from build123d import *

# Parameters (mm, degrees)
F0_R     = 8.5
F1_DEPTH = 2.75
F2_R     = 3.83
F3_DEPTH = 3.6
F4_R     = 2.1875
F5_DEPTH = 3.2
F6_R     = 0.5


with BuildPart() as f1:
    # F0 (on Top) → F1 (new body)
    with BuildSketch(Plane.XY):
        Circle(F0_R)
    extrude(amount=F1_DEPTH)

    # F2 (on face) → F3 (join)
    with BuildSketch(Plane.XY.offset(2.75)):
        Circle(F2_R)
    extrude(amount=F3_DEPTH)

    # F4 (on face) → F5 (cut)
    with BuildSketch(Plane.XY.offset(6.35)):
        Circle(F4_R)
    extrude(amount=-F5_DEPTH, mode=Mode.SUBTRACT)

    # F6
    f6_edges = [f1.edges().sort_by_distance(p)[0] for p in [
        (-8.5, 0, 0),
    ]]
    fillet(f6_edges, radius=F6_R)


solid = f1.part
Model file for the job. Use its own axes, mm. A direction names the side the tool comes from. Coordinates: 2 decimals unless noted, no trailing zeros. Loops run counter-clockwise (first coordinate to the right, second up) from the corner with the lowest first, then second, coordinate; pieces in that order, holes last. Notation, with made-up numbers: (-21.5, 81.25) -> (13.5, 81.25) arc R14 ccw to (13.5, 106.25) -> close; hole circle Ø5 at (61, 57). An arc over 180 degrees is marked (long way). Use one line per item in the form item = value. Start each with the question number.
(1) Probe probe 1 along Y at (x, z) = (0, 4.1); probe 2 along Z at (x, y) = (-2.75, 6.25); probe 3 along X at (y, z) = (1.5, 3.75). List the from-to ranges inside material, lowest first. Write a range as from..to.
(2) Tool access for faces 4 (the flat face through (0, 0, 0)), 5 (the flat face through (4, -2, 2.75)): list every direction of +Z, -Z, +X, -X, +Y, -Y with a clear straight run to the whole face (end or side of a thin tool).
(3) Flat gauge pins, fed straight in: pin 1 (3 mm diameter, centred on y = 2.5, z = 4, fed in from -X); pin 2 (1.3 mm diameter, centred on x = -0.5, y = 0.5, fed in from +Z); pin 3 (2 mm diameter, centred on x = 0, z = 5, fed in from +Y). Where does each tip first touch, or does it go through?
(4) Pull direction Y, two halves, no side cores. Call faces 1 (the cylindrical face through (-1.736, -1.331, 4.772)), 2 (the cylindrical face through (-0.499, 3.797, 4.525)), 3 (the flat face through (2, -2, 6.35)): pulls with the +Y half, pulls with the -Y half, needs draft (parallel to the pull), parting line crosses it, or undercut.
(5) Cut at C-C on z = 4.75. Give the cut face in (x, y) (1 decimal).
(6) Cut at A-A on x = 0. Give the cut face in (y, z).
Values:
q1.probe_1 = -3.83..-2.19, 2.19..3.83
q1.probe_2 = 0..2.75
q1.probe_3 = -3.52..-1.59, 1.59..3.52
q2.face_4 = -Z, +X, -X, +Y, -Y
q2.face_5 = +Z
q3.pin_1 = -8.33
q3.pin_2 = 3.15
q3.pin_3 = 3.83
q4.face_1 = undercut
q4.face_2 = parting line crosses it
q4.face_3 = needs draft
q5.outline = circle Ø7.7 at (0, 0); hole circle Ø4.4 at (0, 0)
q6.outline = (-8.5, 0.5) arc R0.5 ccw to (-8, 0) -> (8, 0) arc R0.5 ccw to (8.5, 0.5) -> (8.5, 2.75) -> (3.83, 2.75) -> (3.83, 6.35) -> (2.19, 6.35) -> (2.19, 3.15) -> (-2.19, 3.15) -> (-2.19, 6.35) -> (-3.83, 6.35) -> (-3.83, 2.75) -> (-8.5, 2.75) -> close
